Design review of the part built by this model. Coordinates are the model's own, in mm. A direction names the side the tool comes from. Coordinates: 2 decimals unless noted, no trailing zeros. Loops run counter-clockwise (first coordinate to the right, second up) from the corner with the lowest first, then second, coordinate; pieces in that order, holes last. Notation, with made-up numbers: M -5.5,51 L 32.5,51 A26 ccw 32.5,68 Z; hole C 2,64 d1. An arc over 180 degrees is marked long. Answer as a JSON object with one key per item and string values. Group by question number.
1. To check wall thickness, follow probe 1 along X at (y, z) = (-1, 0); probe 2 along X at (y, z) = (4.8, -1.25); probe 3 along Z at (x, y) = (-16.3, 1.95). State the ranges of each line that lie inside material, in increasing order.
2. Draft analysis for pull direction X (two halves, no side actions). For faces 5 (the cylindrical face through (4.722, 7.67, 1.107)), 6 (the cylindrical face through (-2.2, 11.5, 0.1)), 7 (the cylindrical face through (6.473, 8.232, -5.514)), state which applies: +X half, -X half, draft (parallel to the pull), parting line (faces both ways), or undercut.
3. Consider section D-D (x = 15.5). State the section outline as (y, z) points.
4. Consider section C-C (z = -5.5). State the section outline as (x, y) points.
5. Consider section A-A (x = 0). State the section outline as (y, z) points.
6. Machinability: for faces 1 (the flat face through (10.8, 8, 0.1)), 2 (the flat face through (8, -1, 2.825)), 3 (the cylindrical face through (10.45, 6.03, -7.93)), 4 (the cylindrical face through (10.48, 6.03, 7.9)), which of the approach directions +Z, -Z, +X, -X, +Y, -Y give a long, thin tool a straight path to every point of the face, cutting with its end or side? Answer none if there is none.
7. Insertion check: pin 1 (1.5 mm diameter, centred on y = 7, z = 6, fed in from +X); pin 2 (3 mm diameter, centred on x = -14, z = 0.5, fed in from +Y); pin 3 (5 mm diameter, centred on x = 15.5, z = 5.5, fed in from +Y). Each pin has a flat end and moves straight along its axis. Give the tip position at first contact, or say it passes through.
8. Consider section B-B (y = -0.75). State the section outline as (x, z) points (3 decimals).
from build123d import *

# Parameters (mm, degrees)
BOSS_EXTRUDE1_DEPTH     = 8.5
CUT_EXTRUDE1_DEPTH      = 2
CUT_EXTRUDE1_DEPTH_BACK = 26.602245995
SKETCH2_R               = 2.75
CUT_EXTRUDE2_DEPTH      = 2
CUT_EXTRUDE2_DEPTH_BACK = 0.25
SKETCH2_3_R             = 5
SKETCH2_3_R_2           = 2.75
SKETCH3_R               = 1.75
CUT_EXTRUDE3_DEPTH      = 28.391148205
SKETCH3_3_R             = 3
SKETCH3_3_R_2           = 1.75
CUT_EXTRUDE4_DEPTH      = 5.85
FILLET1_R               = 2
FILLET2_R               = 2
CUT_EXTRUDE5_DEPTH      = 2


with BuildPart() as part:
    # Sketch1 → Boss-Extrude1 (new, symmetric)
    with BuildSketch(Plane.XY):
        with BuildLine():
            Line((11.05, 4), (3.970201506, 4))
            ThreePointArc((3.970201506, 4), (-3.590264914, 6.674165907), (2.926174978, 2))
            Line((2.926174978, 2), (22.05, 2))
            Line((22.05, 2), (22.05, -2))
            Line((22.05, -2), (-22.05, -2))
            Line((-22.05, -2), (-22.05, 2))
            Line((-22.05, 2), (-9.85, 2))
            ThreePointArc((-9.85, 2), (-7.870101013, 2.820101013), (-7.05, 4.8))
            ThreePointArc((-7.05, 4.8), (-1.645444408, 11.655290855), (6.281918497, 8))
            Line((6.281918497, 8), (11.05, 8))
            Line((11.05, 8), (11.05, 4))
        make_face()
    extrude(amount=BOSS_EXTRUDE1_DEPTH, both=True)

    # Sketch2 → Cut-Extrude1 (cut, two sides: drawn at the far end of the back side and taken through both)
    with BuildSketch(Plane(origin=(0, 2, 0), x_dir=(1, 0, 0), z_dir=(0, 1, 0)).offset(-CUT_EXTRUDE1_DEPTH_BACK)):
        with Locations(Location((16.3, 0, 0), (0, 0, 180))):
            Circle(SKETCH2_R)
        with Locations(Location((-16.3, 0, 0), (0, 0, 180))):
            Circle(SKETCH2_R)
    extrude(amount=CUT_EXTRUDE1_DEPTH + CUT_EXTRUDE1_DEPTH_BACK, mode=Mode.SUBTRACT)

    # Sketch2<3> → Cut-Extrude2 (cut, two sides: drawn at the far end of the back side and taken through both)
    # profile 1 of 2: a face of its own
    with BuildSketch(Plane(origin=(0, 2, 0), x_dir=(1, 0, 0), z_dir=(0, 1, 0)).offset(-CUT_EXTRUDE2_DEPTH_BACK)):
        with Locations(Location((16.3, 0, 0), (0, 0, 180))):
            Circle(SKETCH2_3_R)
        with Locations(Location((16.3, 0, 0), (0, 0, 180))):
            Circle(SKETCH2_3_R_2, mode=Mode.SUBTRACT)
    # profile 2 of 2: a face of its own
    with BuildSketch(Plane(origin=(0, 2, 0), x_dir=(1, 0, 0), z_dir=(0, 1, 0)).offset(-CUT_EXTRUDE2_DEPTH_BACK)):
        with Locations(Location((-16.3, 0, 0), (0, 0, 180))):
            Circle(SKETCH2_3_R)
        with Locations(Location((-16.3, 0, 0), (0, 0, 180))):
            Circle(SKETCH2_3_R_2, mode=Mode.SUBTRACT)
    extrude(amount=CUT_EXTRUDE2_DEPTH + CUT_EXTRUDE2_DEPTH_BACK, mode=Mode.SUBTRACT)

    # Sketch3 → Cut-Extrude3 (cut, through all)
    with BuildSketch(Plane(origin=(0, 11.85, 0), x_dir=(1, 0, 0), z_dir=(0, 1, 0))):
        with Locations(Location((7.510100753, 0, 0), (0, 0, 225.426920251))):
            Circle(SKETCH3_R)
    extrude(amount=-CUT_EXTRUDE3_DEPTH, mode=Mode.SUBTRACT)

    # Sketch3<3> → Cut-Extrude4 (cut)
    # profile 1 of 2: a face of its own
    with BuildSketch(Plane(origin=(0, 11.85, 0), x_dir=(1, 0, 0), z_dir=(0, 1, 0))):
        with Locations(Location((7.510100753, 0, 0), (0, 0, 245.83322212))):
            Circle(SKETCH3_3_R)
        with Locations(Location((7.510100753, 0, 0), (0, 0, 180))):
            Circle(SKETCH3_3_R_2, mode=Mode.SUBTRACT)
    # profile 2 of 2: a face of its own
    with BuildSketch(Plane(origin=(0, 11.85, 0), x_dir=(1, 0, 0), z_dir=(0, 1, 0))):
        with Locations(Location((7.510100753, 0, 0), (0, 0, 180))):
            Circle(SKETCH3_3_R_2)
    extrude(amount=-CUT_EXTRUDE4_DEPTH, mode=Mode.SUBTRACT)

    # Fillet1
    fillet1_edges = [part.edges().sort_by_distance(p)[0] for p in [
        (22.05, 0, 8.5),
        (22.05, 0, -8.5),
        (-22.05, 0, -8.5),
        (-22.05, 0, 8.5),
    ]]
    fillet(fillet1_edges, radius=FILLET1_R)

    # Fillet2
    # the kernel refuses this fillet: 2 mm, written as the material it adds along each edge
    with BuildSketch(Plane(origin=(6.281918497, 8, -0.075436901), x_dir=(1, 0, 0), z_dir=(0, 0, 1))) as fillet2_piece_1_section:
        with BuildLine():
            CenterArc((1.125003941, 2), FILLET2_R, 215.07061915, 54.92938085)
            ThreePointArc((-0.511884995, 0.850828729), (-0.240944724, 0.434437491), (0, 0))
            Line((0, 0), (1.125003941, 0))
        make_face()
    fillet2_piece_1 = extrude(amount=8.575436901, mode=Mode.PRIVATE)
    fillet2_piece_1 = fillet2_piece_1 - Plane(origin=(7.510100753, 8.184515376, 0), x_dir=(-0.4093940854484991, 0, 0.9123576507049125), z_dir=(0, 1, 0)) * Cylinder(3, 22, mode=Mode.PRIVATE)
    add(fillet2_piece_1)
    with BuildSketch(Plane(origin=(6.281918497, 8, -8.5), x_dir=(1, 0, 0), z_dir=(0, 0, 1))) as fillet2_piece_2_section:
        with BuildLine():
            CenterArc((1.125003941, 2), FILLET2_R, 215.07061915, 54.92938085)
            ThreePointArc((-0.511884995, 0.850828729), (-0.240944724, 0.434437491), (0, 0))
            Line((0, 0), (1.125003941, 0))
        make_face()
    fillet2_piece_2 = extrude(amount=8.575436901, mode=Mode.PRIVATE)
    fillet2_piece_2 = fillet2_piece_2 - Plane(origin=(7.510100753, 8.184515325, 0), x_dir=(-0.4093940854484991, 0, 0.9123576507049125), z_dir=(0, 1, 0)) * Cylinder(3, 22, mode=Mode.PRIVATE)
    add(fillet2_piece_2)
    # the kernel refuses this fillet: 2 mm, written as the material it takes off along each edge
    with BuildSketch(Plane(origin=(11.05, 13, -8.5), x_dir=(-1, 0, 0), z_dir=(0, -1, 0))) as fillet2_2_piece_1_section:
        with BuildLine():
            CenterArc((FILLET2_R, -FILLET2_R), FILLET2_R, 90, 90)
            Line((0, -FILLET2_R), (0, 0))
            Line((0, 0), (FILLET2_R, 0))
        make_face()
    fillet2_2_piece_1 = extrude(amount=14, mode=Mode.PRIVATE)
    fillet2_2_piece_1 = split(fillet2_2_piece_1, bisect_by=Plane(origin=(10.603264122, 2, -8.053264122), z_dir=(0, 1, 0)), keep=Keep.TOP, mode=Mode.PRIVATE)
    add(fillet2_2_piece_1, mode=Mode.SUBTRACT)
    with BuildSketch(Plane(origin=(11.05, 13, 8.5), x_dir=(-1, 0, 0), z_dir=(0, -1, 0))) as fillet2_2_piece_2_section:
        with BuildLine():
            CenterArc((FILLET2_R, FILLET2_R), FILLET2_R, 180, 90)
            Line((0, FILLET2_R), (0, 0))
            Line((0, 0), (FILLET2_R, 0))
        make_face()
    fillet2_2_piece_2 = extrude(amount=14, mode=Mode.PRIVATE)
    fillet2_2_piece_2 = split(fillet2_2_piece_2, bisect_by=Plane(origin=(10.603264122, 2, 8.053264122), z_dir=(0, 1, 0)), keep=Keep.TOP, mode=Mode.PRIVATE)
    add(fillet2_2_piece_2, mode=Mode.SUBTRACT)

    # Sketch4 → Cut-Extrude5 (cut)
    with BuildSketch(Plane.XZ.offset(2)):
        Polygon((10.772129774, 0), (9.141115264, 2.825), (5.879086243, 2.825), (4.248071732, 0), (5.879086243, -2.825), (9.141115264, -2.825), align=None)
    extrude(amount=-CUT_EXTRUDE5_DEPTH, mode=Mode.SUBTRACT)


solid = part.part
Findings below:
{
 "1": {"probe 1": "x = -22.05 to -19.05, -13.55 to 4.25, 10.77 to 13.55, 19.05 to 22.05", "probe 2": "x = -7.05 to -4.05, 4.05 to 6.29, 8.73 to 11.05", "probe 3": "z = -8.5 to -5, 5 to 8.5"},
 "2": {"face 5": "undercut", "face 6": "parting line", "face 7": "+X half"},
 "3": {"outline": "M -2,-8.5 L 2,-8.5 L 2,-4.94 L 1.75,-4.94 L 1.75,-2.63 L -2,-2.63 Z; M -2,2.63 L 1.75,2.63 L 1.75,4.94 L 2,4.94 L 2,8.5 L -2,8.5 Z"},
 "4": {"outline": "M -22.05,-2 L 22.05,-2 L 22.05,2 L 2.93,2 A4.05 cw long 3.97,4 L 11.05,4 L 11.05,8 L 7.41,8 A2 cw 5.77,8.85 A7.05 ccw -7.05,4.8 A2.8 cw -9.85,2 L -22.05,2 Z"},
 "5": {"outline": "M -2,-8.5 L 0.75,-8.5 L 0.75,8.5 L -2,8.5 Z; M 8.85,-8.5 L 11.85,-8.5 L 11.85,8.5 L 8.85,8.5 Z"},
 "6": {"face 1": "+Z, -Z, +X, +Y", "face 2": "-Y", "face 3": "-Z, +X, +Y", "face 4": "+Z, +X, +Y"},
 "7": {"pin 1": "stops at x = 11.05", "pin 2": "stops at y = 1.75", "pin 3": "stops at y = 2"},
 "8": {"outline": "M -22.05,-6.5 A2 ccw -20.05,-8.5 L 20.05,-8.5 A2 ccw 22.05,-6.5 L 22.05,6.5 A2 ccw 20.05,8.5 L -20.05,8.5 A2 ccw -22.05,6.5 Z; hole C -16.3,0 d5.5; hole M 4.248,0 L 5.879,-2.825 L 9.141,-2.825 L 10.772,0 L 9.141,2.825 L 5.879,2.825 Z; hole C 16.3,0 d5.5"}
}
